from build123d import *

# Parameters (mm, degrees)
SKETCH1_W                                = 84
SKETCH1_H                                = 84
BOSS_EXTRUDE1_DEPTH                      = 6
SKETCH2_R                                = 1.5
CUT_EXTRUDE1_DEPTH                       = 119.94536561
SKETCH5_W                                = 50.5
SKETCH5_H                                = 34
BOSS_EXTRUDE2_DEPTH                      = 22
SKETCH6_W                                = 44.5
SKETCH6_H                                = 28
CUT_EXTRUDE5_DEPTH                       = 25
FILLET1_R                                = 3
SKETCH8_R                                = 12.5
CUT_EXTRUDE6_DEPTH                       = 10
CUT_EXTRUDE7_DEPTH                       = 123.049170419
CUT_EXTRUDE7_DEPTH_BACK                  = 123.049170419
SKETCH9_W                                = 84
SKETCH9_H                                = 8
CUT_EXTRUDE8_DEPTH                       = 3
MIRROR1_AT_THE_SECOND_PLANE_COPY_1_DEPTH = 3
SKETCH13_R                               = 5.5
CUT_EXTRUDE9_DEPTH                       = 14
CUT_EXTRUDE10_DEPTH                      = 10
CUT_EXTRUDE11_DEPTH                      = 10
BOSS_EXTRUDE3_DEPTH                      = 3
CUT_EXTRUDE14_DEPTH                      = 4
SKETCH20_W                               = 13.564659966
SKETCH20_H                               = 7
CUT_EXTRUDE15_DEPTH                      = 4


with BuildPart() as part:
    # Sketch1 → Boss-Extrude1 (new body)
    with BuildSketch(Plane(origin=(0, 0, 0), x_dir=(1, 0, 0), z_dir=(0, 1, 0))):
        with Locations((42, 42)):
            Rectangle(SKETCH1_W, SKETCH1_H)
    extrude(amount=BOSS_EXTRUDE1_DEPTH)

    # Sketch2 → Cut-Extrude1 (cut, through all)
    with BuildSketch(Plane(origin=(0, 6, 0), x_dir=(1, 0, 0), z_dir=(0, 1, 0))):
        with Locations(Location((6, 72, 0), (0, 0, 270))):
            Circle(SKETCH2_R)
        with Locations(Location((6, 12, 0), (0, 0, 270))):
            Circle(SKETCH2_R)
        with Locations(Location((78, 12, 0), (0, 0, 270))):
            Circle(SKETCH2_R)
        with Locations(Location((78, 72, 0), (0, 0, 270))):
            Circle(SKETCH2_R)
    extrude(amount=-CUT_EXTRUDE1_DEPTH, mode=Mode.SUBTRACT)

    # Sketch5 → Boss-Extrude2 (add)
    with BuildSketch(Plane(origin=(0, 6, 0), x_dir=(1, 0, 0), z_dir=(0, 1, 0))):
        with Locations((34.5, 17)):
            Rectangle(SKETCH5_W, SKETCH5_H)
    extrude(amount=BOSS_EXTRUDE2_DEPTH)

    # Sketch6 → Cut-Extrude5 (cut)
    with BuildSketch(Plane(origin=(0, 28, 0), x_dir=(1, 0, 0), z_dir=(0, 1, 0))):
        with Locations((34.5, 17)):
            Rectangle(SKETCH6_W, SKETCH6_H)
    extrude(amount=-CUT_EXTRUDE5_DEPTH, mode=Mode.SUBTRACT)

    # Fillet1
    fillet1_edges = [part.edges().sort_by_distance(p)[0] for p in [
        (59.75, 17, -34),
        (9.25, 17, -34),
        (9.25, 17, 0),
        (59.75, 17, 0),
    ]]
    fillet(fillet1_edges, radius=FILLET1_R)

    # Sketch8 → Cut-Extrude6 (cut)
    with BuildSketch(Plane.XY):
        with Locations((42.25, 13.5)):
            Circle(SKETCH8_R)
    extrude(amount=-CUT_EXTRUDE6_DEPTH, mode=Mode.SUBTRACT)

    # Sketch9 → Cut-Extrude7 (cut, two sides: drawn at the far end of the back side and taken through both)
    with BuildSketch(Plane.XY.offset(-CUT_EXTRUDE7_DEPTH_BACK)):
        with Locations((42, 24)):
            Rectangle(SKETCH9_W, SKETCH9_H)
    extrude(amount=CUT_EXTRUDE7_DEPTH + CUT_EXTRUDE7_DEPTH_BACK, mode=Mode.SUBTRACT)

    # Sketch11 → Cut-Extrude8 (cut)
    with BuildSketch(Plane.XZ):
        Polygon((3, -9), (13, -9), (13, -15), (8, -21), (3, -21), align=None)
    cut_extrude8 = extrude(amount=-CUT_EXTRUDE8_DEPTH, mode=Mode.SUBTRACT)

    # Mirror1: Cut-Extrude8 across plane
    add(cut_extrude8.mirror(Plane.XY.offset(-42)), mode=Mode.SUBTRACT)

    # Mirror1 at the second plane: Cut-Extrude8 across plane
    add(cut_extrude8.mirror(Plane.ZY.offset(-42)), mode=Mode.SUBTRACT)

    # Mirror1 at the second plane copy 1 sketc → Mirror1 at the second plane copy 1 (cut)
    with BuildSketch(Plane(origin=(84, 0, -84), x_dir=(-1, 0, 0), z_dir=(0, -1, 0))):
        Polygon((3, -9), (13, -9), (13, -15), (8, -21), (3, -21), align=None)
    extrude(amount=-MIRROR1_AT_THE_SECOND_PLANE_COPY_1_DEPTH, mode=Mode.SUBTRACT)

    # Sketch13 → Cut-Extrude9 (cut)
    with BuildSketch(Plane(origin=(0, 20, 0), x_dir=(1, 0, 0), z_dir=(0, 1, 0))):
        with Locations((6, 12)):
            Circle(SKETCH13_R)
    extrude(amount=-CUT_EXTRUDE9_DEPTH, mode=Mode.SUBTRACT)

    # Sketch14 → Cut-Extrude10 (cut)
    with BuildSketch(Plane.XY):
        Polygon((29.75, 13.5), (29.75, 20), (31.572921748, 20), align=None)
    extrude(amount=-CUT_EXTRUDE10_DEPTH, mode=Mode.SUBTRACT)

    # Sketch15 → Cut-Extrude11 (cut)
    with BuildSketch(Plane.XY):
        Polygon((54.75, 20), (54.75, 13.5), (52.927078252, 20), align=None)
    extrude(amount=-CUT_EXTRUDE11_DEPTH, mode=Mode.SUBTRACT)

    # Sketch17 → Boss-Extrude3 (add)
    with BuildSketch(Plane.XZ):
        Polygon((8.833333333, -9), (8.833333333, -20), (13, -15), (13, -9), align=None)
    extrude(amount=-BOSS_EXTRUDE3_DEPTH)

    # Sketch18 → Cut-Extrude14 (cut)
    with BuildSketch(Plane(origin=(0, 3, 0), x_dir=(1, 0, 0), z_dir=(0, 1, 0))):
        Polygon((35.467670017, 3), (35.467670017, 10), (49.032329983, 10), (49.032329983, 3), (56.75, 3), (56.75, 31), (12.25, 31), (12.25, 3), align=None)
    extrude(amount=-CUT_EXTRUDE14_DEPTH, mode=Mode.SUBTRACT)

    # Sketch20 → Cut-Extrude15 (cut)
    with BuildSketch(Plane.XZ):
        with Locations((42.25, -6.5)):
            Rectangle(SKETCH20_W, SKETCH20_H)
    extrude(amount=-CUT_EXTRUDE15_DEPTH, mode=Mode.SUBTRACT)


solid = part.part
Geometry: final body of the model. Coordinates: model frame, mm. A direction names the side the tool comes from. Round coordinates to 2 decimals unless told otherwise and drop trailing zeros. Loops run counter-clockwise (first coordinate to the right, second up) from the corner with the lowest first, then second, coordinate; pieces in that order, holes last. Notation, with made-up numbers: (5, -1) - (31, -1) arc R16 ccw to (31, 3) - close; hole circle Ø3 at (-19.75, -26). An arc over 180 degrees is marked (long way). Write each question's results on one line, items separated by ' | '. Start each with the question number.
1) Cut plane C-C on z = -72. Return loops of the section in (x, y), then the cut area to 3 significant figures.
2) Line query: probe 1 along X at (y, z) = (4.75, -12); probe 2 along X at (y, z) = (2.5, -15); probe 3 along X at (y, z) = (4.2, -72). Output: solid intervals per line, ascending. Write a range as [from, to].
3) First-contact query: P1, Ø4, axis at x = 42, y = 15, coming from the +Z side; P2, Ø12, axis at x = 13.5, y = 16, coming from the -Z side; P3, Ø1, axis at x = 22, z = -73, coming from the +Y side. Flat tips, straight axial feed; report the tip coordinate or a pass-through.
4) Mould query, pull axis X, two halves, no side actions, for faces 1 (the face through (41, 0, -51)), 2 (the face through (8, 3, -69)), 3 (the face through (9.25, 13, -5)). Classes: released by +X, released by -X, zero draft, split by the parting line, or undercut.
5) Cut plane B-B on z = -26. Return loops of the section in (x, y), then the cut area to 3 significant figures.
6) Cut plane A-A on x = 42.25. Return loops of the section in (y, z).
7) Access query for faces 4 (the face through (11.5, 13.1, -11.9)), 5 (the face through (29.75, 17, -1)), 6 (the face through (56.75, 10, -17)), 7 (the face through (76, 3, -15)), 8 (the face through (59.75, 13, -17)). Directions: +Z, -Z, +X, -X, +Y, -Y. A direction counts if a zero-diameter tool reaches every point of the face in a straight line with its end or side. Return the directions, or none.
8) Cut plane D-D on x = 78. Return loops of the section in (y, z), then the cut area to 3 significant figures.
Verdict:
1) outline: (0, 0) - (3, 0) - (3, 3) - (4.5, 3) - (4.5, 6) - (0, 6) - close; (7.5, 3) - (13, 3) - (13, 0) - (71, 0) - (71, 3) - (76.5, 3) - (76.5, 6) - (7.5, 6) - close; (79.5, 3) - (81, 3) - (81, 0) - (84, 0) - (84, 6) - (79.5, 6) - close | area: 426 mm2
2) probe 1: x = [0, 4.5], [7.5, 12.25], [56.75, 76.5], [79.5, 84] | probe 2: x = [0, 3], [8.83, 12.25], [56.75, 71], [81, 84] | probe 3: x = [0, 4.5], [7.5, 76.5], [79.5, 84]
3) P1: stops at z = -31 | P2: stops at z = -34 | P3: stops at y = 6
4) face 1: zero draft | face 2: undercut | face 3: released by -X
5) outline: (0, 0) - (12.25, 0) - (12.25, 20) - (9.25, 20) - (9.25, 6) - (0, 6) - close; (56.75, 0) - (84, 0) - (84, 6) - (59.75, 6) - (59.75, 20) - (56.75, 20) - close | area: 321 mm2
6) outline: (0, -84) - (6, -84) - (6, -34) - (20, -34) - (20, -31) - (0, -31) - close; (0, -3) - (1, -3) - (1, 0) - (0, 0) - close
7) face 4: -X, +Y | face 5: +Z, +Y | face 6: +Y, -Y | face 7: -Y | face 8: +Z, -Z, +X, +Y
8) outline: (0, -84) - (6, -84) - (6, -73.5) - (3, -73.5) - (3, -75) - (0, -75) - close; (0, -63) - (3, -63) - (3, -70.5) - (6, -70.5) - (6, -13.5) - (3, -13.5) - (3, -21) - (0, -21) - close; (0, -9) - (3, -9) - (3, -10.5) - (6, -10.5) - (6, 0) - (0, 0) - close | area: 414 mm2
